from build123d import *

# Parameters (mm, degrees)
F1_DEPTH = 38.1
F2_R     = 5.08


with BuildPart() as f1:
    # F0 (on Top) → F1 (new body)
    with BuildSketch(Plane.XY):
        with BuildLine():
            Line((-38.1, 0), (38.1, 0))
            ThreePointArc((38.1, 0), (0, 38.1), (-38.1, 0))
        make_face()
    extrude(amount=F1_DEPTH)

    # F2
    f2_edges = [f1.edges().sort_by_distance(p)[0] for p in [
        (0, 38.1, 38.1),
        (38.1, 0, 19.05),
        (-38.1, 0, 19.05),
        (0, 38.1, 0),
    ]]
    fillet(f2_edges, radius=F2_R)


solid = f1.part
For this review, take the finished solid that the model builds, in its own axes (mm). Give positions to 0.01 mm unless a question says otherwise; leave off trailing zeros. Order: outer loops, then holes, each group sorted by start corner. A loop starts at its lowest first (then second) coordinate and runs counter-clockwise, first axis right, second up. Notation, with made-up numbers: (-6, 50) -> (43, 50) arc R14 cw to (43, 72) -> close; hole circle Ø4 at (-8, -3.5). An arc over 180 degrees is marked (long way). Write item = value, one per line.
1) Insertion check: pin 1 (6 mm diameter, centred on x = -28.5, y = 8, fed in from -Z); pin 2 (3 mm diameter, centred on x = 10, z = 29.5, fed in from +Y); pin 3 (6 mm diameter, centred on y = 12.5, z = 8.5, fed in from +X); pin 4 (1.5 mm diameter, centred on x = -4.5, z = 11.5, fed in from +Y) (3 decimals). Each pin has a flat end and moves straight along its axis. Give the tip position at first contact, or say it passes through.
Findings:
pin_1 = 0
pin_2 = 37.14
pin_3 = 36.9
pin_4 = 37.915
2) We need section B-B, the plane z = 34.5. Give the boundary of the cut face in (x, y), and give its area (3 significant figures).
Findings:
outline = (-37.64, 4.26) arc R5.08 ccw to (-32.63, 0) -> (32.63, 0) arc R5.08 ccw to (37.64, 4.26) arc R37.88 ccw to start
area = 2,240 mm^2
3) To check wall thickness, follow L1, parallel to X at y = 19, z = 22.5; L2, parallel to X at y = 18, z = 17.5; L3, parallel to Y at x = 11.5, z = 24. State the ranges of each line that lie inside material, in increasing order. Write a range as from..to.
Findings:
L1 = -33.02..33.02
L2 = -33.58..33.58
L3 = 0..36.32
4) We need section A-A, the plane z = 14.5. Give the boundary of the cut face in (x, y).
Findings:
outline = (-37.65, 5.86) arc R5.08 ccw to (-32.63, 0) -> (32.63, 0) arc R5.08 ccw to (37.65, 5.86) arc R38.1 ccw to start
